Drawing for the job (mm, zero at the part's lowest x, y, z). A direction names the side the tool comes from. Give positions to 0.01 mm unless a question says otherwise; leave off trailing zeros. Order: outer loops, then holes, each group sorted by start corner. A loop starts at its lowest first (then second) coordinate and runs counter-clockwise, first axis right, second up. Notation, with made-up numbers: (40, 70.5) - (75, 70.5) arc R32 cw to (75, 103.5) - close; hole circle Ø3 at (73, 34.5). An arc over 180 degrees is marked (long way). Use a Markdown table: item, result. Add a question column.
(1) Slice it at D-D (y = 14). Write the cut outline in (x, z).
(2) Slice it at C-C (z = 5). Write the cut outline in (x, y) (1 decimal).
(3) Mould opens along X. For the marked faces 4, 5 and 6 say: +X half, -X half, draft (parallel to the pull), parting line (faces both ways), or undercut.
(4) Slice it at B-B (x = 7). Write the cut outline in (y, z) (1 decimal).
(5) Wall check: line 1 (X direction, y = 3.25, z = 5); line 2 (Y direction, x = 5.25, z = 7) (1 decimal); line 3 (Y direction, x = 5, z = 1.5) (1 decimal). Give the ranges that are in metal, low to high.
(6) Flat gauge pins, fed straight in: pin 1 (6 mm diameter, centred on x = 6.5, z = 1.5, fed in from -Y); pin 2 (1.5 mm diameter, centred on x = 8.5, z = 6, fed in from -Y) (1 decimal); pin 3 (2 mm diameter, centred on y = 4, z = 8.5, fed in from -X). Where does each tip first touch, or does it go through?
(7) Slice it at A-A (y = 7). Write the cut outline in (x, z).
(8) Which spindle directions (+Z, -Z, +X, -X, +Y, -Y) get a long thin tool onto all of the face, cutting with end or side? Do the marked faces 1, 2 and 3. Say none if no direction does.
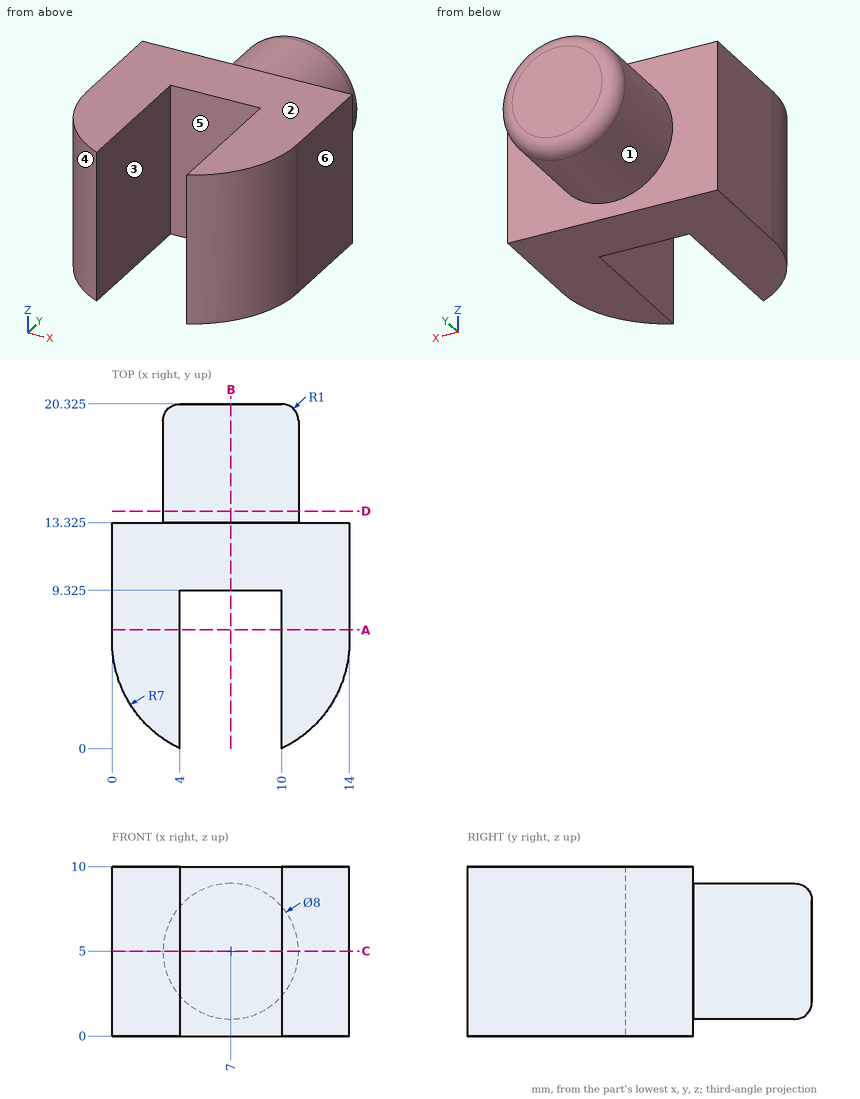
Solution:
| question | item | result |
|---|---|---|
| 1 | outline | circle Ø8 at (7, 5) |
| 2 | outline | (0, 6.3) arc R7 ccw to (4, 0) - (4, 9.3) - (10, 9.3) - (10, 0) arc R7 ccw to (14, 6.3) - (14, 13.3) - (11, 13.3) - (11, 19.3) arc R1 ccw to (10, 20.3) - (4, 20.3) arc R1 ccw to (3, 19.3) - (3, 13.3) - (0, 13.3) - close |
| 3 | face 4 | -X half |
| 3 | face 5 | undercut |
| 3 | face 6 | +X half |
| 4 | outline | (9.3, 0) - (13.3, 0) - (13.3, 1) - (19.3, 1) arc R1 ccw to (20.3, 2) - (20.3, 8) arc R1 ccw to (19.3, 9) - (13.3, 9) - (13.3, 10) - (9.3, 10) - close |
| 5 | line 1 | 0.71 to 4, 10 to 13.29 |
| 5 | line 2 | 9.3 to 20.3 |
| 5 | line 3 | 9.3 to 13.3 |
| 6 | pin 1 | y = 0 |
| 6 | pin 2 | y = 9.3 |
| 6 | pin 3 | x = 0.13 |
| 7 | outline | (0, 0) - (4, 0) - (4, 10) - (0, 10) - close; (10, 0) - (14, 0) - (14, 10) - (10, 10) - close |
| 8 | face 1 | +Y |
| 8 | face 2 | +Z, +X, -X, +Y, -Y |
| 8 | face 3 | +Z, -Z, -Y |
